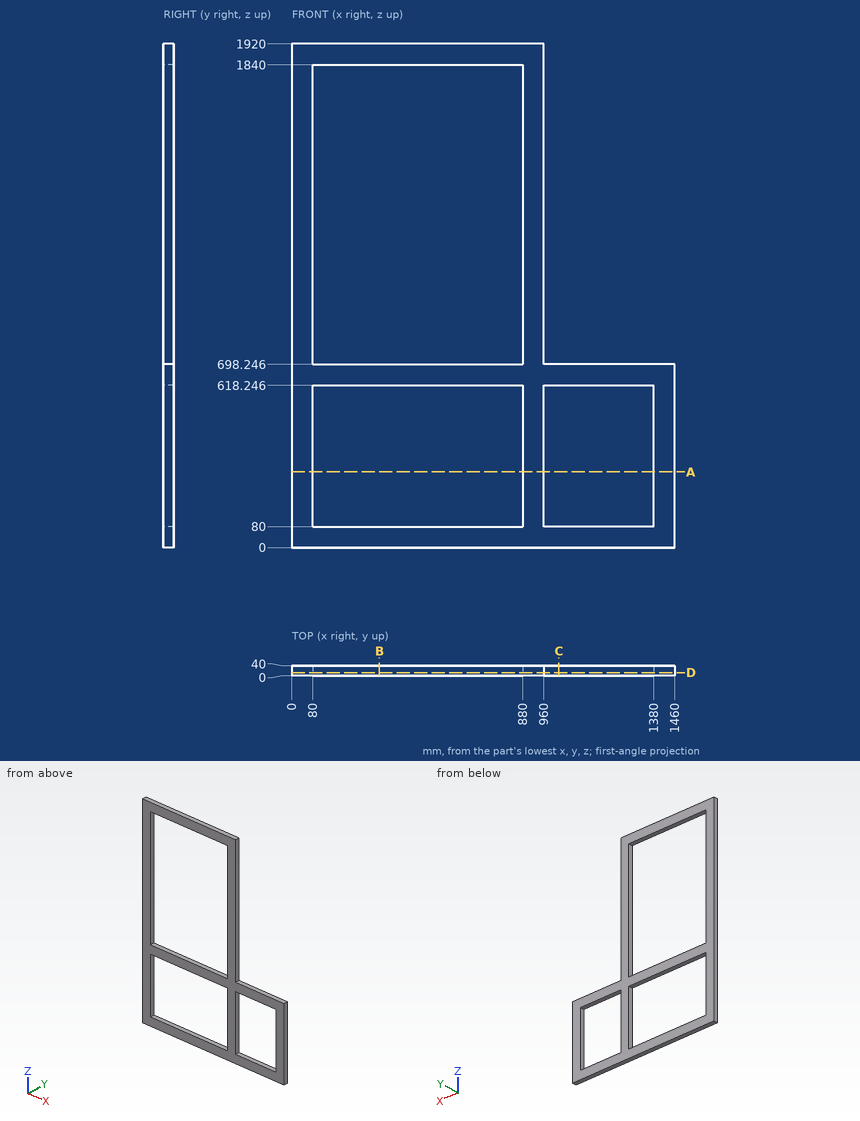
Study the drawing (mm; zero at the part's minimum x, y, z) and answer. Round coordinates to 2 decimals unless told otherwise and drop trailing zeros. Write each loop counter-clockwise with the first axis right and the second up, starting at its lowest first coordinate (ties: lowest second). Pieces come first, ordered by that corner, then holes.
Q1. Find section C-C on x = 1018.5. Determine the outline of the cut face in (y, z).
Values:
outline: (0, 0) - (40, 0) - (40, 80) - (0, 80) - close; (0, 618.25) - (40, 618.25) - (40, 698.25) - (0, 698.25) - close
Q2. Find section B-B on x = 334. Determine the outline of the cut face in (y, z), and give its area (3 significant figures).
Values:
outline: (0, 0) - (40, 0) - (40, 80) - (0, 80) - close; (0, 618.25) - (40, 618.25) - (40, 698.25) - (0, 698.25) - close; (0, 1840) - (40, 1840) - (40, 1920) - (0, 1920) - close
area: 9,600 mm2
Q3. Straight lines are drawn through the part: line 1 (Z direction, x = 587, y = 10.5); line 2 (X direction, y = 14, z = 193); line 3 (Z direction, x = 1123.5, y = 36). For each, find the intervals that lie inside material, in ascending order.
Values:
line 1: z = 0 to 80, 618.25 to 698.25, 1840 to 1920
line 2: x = 0 to 80, 880 to 960, 1380 to 1460
line 3: z = 0 to 80, 618.25 to 698.25
Q4. Find section A-A on z = 288. Determine the outline of the cut face in (x, y).
Values:
outline: (0, 0) - (80, 0) - (80, 40) - (0, 40) - close; (880, 0) - (960, 0) - (960, 40) - (880, 40) - close; (1380, 0) - (1460, 0) - (1460, 40) - (1380, 40) - close
Q5. Flat-ended cylindrical pins translate along their axes: P1, Ø12, axis at y = 33.5, z = 1701, coming from the +X side; P2, Ø12, axis at x = 1084.5, y = 24, coming from the +Z side. Find the tip coordinate at first contact, or state that the pin passes through.
Values:
P1: stops at x = 960
P2: stops at z = 698.25
Q6. Find section D-D on y = 13. Determine the outline of the cut face in (x, z).
Values:
outline: (0, 0) - (1460, 0) - (1460, 698.25) - (960, 698.25) - (960, 1920) - (0, 1920) - close; hole (80, 80) - (880, 80) - (880, 618.25) - (80, 618.25) - close; hole (80, 698.25) - (880, 698.25) - (880, 1840) - (80, 1840) - close; hole (960, 80) - (1380, 80) - (1380, 618.25) - (960, 618.25) - close
